Autodesk Inventor part; units mm, degrees
ref_plane "YZ Plane" through (0, 0, 0) normal (1, 0, 0) x (0, 1, 0)
ref_plane "XZ Plane" through (0, 0, 0) normal (0, 1, 0) x (-1, 0, 0)
ref_plane "XY Plane" through (0, 0, 0) normal (0, 0, 1) x (1, 0, 0)
sketch "Sketch1" plane through (0, 0, 0) normal (1, 0, 0) x (0, 1, 0)
  line L0 (0, 0) -> (46, 0)
  line L1 (46, 0) -> (46, -32)
  line L2 (46, -32) -> (0, -32)
  line L3 (0, -32) -> (0, 0)
  dimension "d0" = 46
  dimension "d1" = 32
extrude "Extrusion1" add sketch "Sketch1" along normal blind 25.2
sketch "Sketch3" plane through (0, 46, 0) normal (0, 1, 0) x (1, 0, 0)
  circle A0 centre (11.23, 13.585) radius 13.2
  line L0 (25.2, 32) -> (25.2, 0)
  line L1 (0, 32) -> (25.2, 32)
  point P0 (0, 0)
  dimension "d4" = 26.4
  dimension "d5" = 13.97
  dimension "d6" = 18.415
extrude "Extrusion2" add sketch "Sketch3" along normal blind 30.8
sketch "Sketch4" plane through (25.2, 0, 0) normal (1, 0, 0) x (0, 0, -1)
  circle A0 centre (7, 39) radius 1.5
  circle A1 centre (25, 39) radius 1.5
  circle A2 centre (6.5, 6) radius 1.5
  circle A3 centre (24.5, 6) radius 1.5
  line L0 (32, 46) -> (0, 46)
  line L1 (32, 0) -> (32, 46)
  point P0 (0, 0)
  dimension "d9" = 3
  dimension "d10" = 3
  dimension "d11" = 3
  dimension "d12" = 3
  dimension "d13" = 7
  dimension "d14" = 7
  dimension "d15" = 18
  dimension "d16" = 33
  dimension "d17" = 33
  dimension "d18" = 18
  dimension "d19" = 7
  dimension "d20" = 7.5
extrude "Extrusion3" cut sketch "Sketch4" against normal blind 5
sketch "Sketch5" plane through (25.2, 0, 0) normal (1, 0, 0) x (0, 0, -1)
  circle A0 centre (15.998, 15) radius 3
  line L0 (32, 0) -> (32, 46)
  line L1 (0, 0) -> (32, 0)
  dimension "d23" = 6
  dimension "d24" = 16.002
  dimension "d25" = 15
extrude "Extrusion4" add sketch "Sketch5" along normal blind 20.5
properties part number "motor"
Model file for the job. Use its own axes, mm. A direction names the side the tool comes from. Round coordinates to 2 decimals unless told otherwise and drop trailing zeros. Write each loop counter-clockwise with the first axis right and the second up, starting at its lowest first coordinate (ties: lowest second). Pieces come first, ordered by that corner, then holes. Notation, with made-up numbers: (23, 20) - (35, 20) arc R19 cw to (35, 24) - close; hole circle Ø6 at (52.5, -33.5). An arc over 180 degrees is marked (long way). Use CSV: the item, a comma, the result in double quotes. Start each with the question number.
Item 1: Two-plate mould, pull along Z, no slides. Class faces 5 (the face through (20.2, 6, -24)), 6 (the face through (35.306, 17.662, -17.382)), 7 (the face through (25.2, 23, -16)): released by +Z, released by -Z, zero draft, split by the parting line, or undercut.
Item 2: Band-saw the part on D-D (z = -24.5). Write the cut outline in (x, y), and give its area (3 significant figures).
Item 3: Band-saw the part on C-C (x = 30). Write the cut outline in (y, z), and give its area (3 significant figures).
Item 4: Tool access for faces 1 (the face through (45.7, 15, -16)), 2 (the face through (22.7, 38.1, -23.8)), 3 (the face through (-1, 46, -14)), 4 (the face through (8.37, 61.18, -26.47)): list every direction of +Z, -Z, +X, -X, +Y, -Y with a clear straight run to the whole face (end or side of a thin tool).
Item 5: Band-saw the part on B-B (z = -15.5). Write the cut outline in (x, y), and give its area (3 significant figures).
Item 6: Pin check, flat tips, straight feed: P1, Ø3.5, axis at y = 6, z = -24.5, coming from the +X side; P2, Ø0.9, axis at y = 6.5, z = -24, coming from the +X side; P3, Ø10, axis at y = 62.5, z = -8, coming from the +X side. Stop position of each tip, or through.
Item 7: Drill centre lines: L1, parallel to Y at x = 22, z = -6; L2, parallel to Y at x = 21, z = -24; L3, parallel to X at y = 16.5, z = -4. Where is each one in solid material? Low to high. Write a range as [from, to].
Item 8: Band-saw the part on A-A (y = 15). Write the cut outline in (x, z), and give its area (3 significant figures).
Checked values:
1,face 5,"undercut"
1,face 6,"split by the parting line"
1,face 7,"zero draft"
2,outline,"(0, 0) - (25.2, 0) - (25.2, 4.5) - (20.2, 4.5) - (20.2, 7.5) - (25.2, 7.5) - (25.2, 37.59) - (20.2, 37.59) - (20.2, 40.41) - (25.2, 40.41) - (25.2, 46) - (18.65, 46) - (18.65, 76.8) - (3.81, 76.8) - (3.81, 46) - (0, 46) - close"
2,area,"1,590 mm²"
3,outline,"circle Ø6 at (15, -16)"
3,area,"28.3 mm²"
4,face 1,"+Z, -Z, +X, +Y, -Y"
4,face 2,"+X"
4,face 3,"+Z, -Z, -X, -Y"
4,face 4,"+Y"
5,outline,"(-1.83, 46) - (0, 46) - (0, 0) - (25.2, 0) - (25.2, 12.04) - (45.7, 12.04) - (45.7, 17.96) - (25.2, 17.96) - (25.2, 46) - (24.29, 46) - (24.29, 76.8) - (-1.83, 76.8) - close"
5,area,"2,090 mm²"
6,P1,"stops at x = 25.2"
6,P2,"stops at x = 20.2"
6,P3,"stops at x = 24.42"
7,L1,"y = [0, 4.59], [7.41, 37.88], [40.12, 76.8]"
7,L2,"y = [0, 4.59], [7.41, 37.88], [40.12, 46]"
7,L3,"x = [0, 25.2]"
8,outline,"(0, -32) - (25.2, -32) - (25.2, -19) - (45.7, -19) - (45.7, -13) - (25.2, -13) - (25.2, 0) - (0, 0) - close"
8,area,"929 mm²"
